Source: CAD feature listing. Evaluate the final solid. Frame: model axes, mm. Face numbers are marked on the shaded views. A direction names the side the tool comes from. Round coordinates to 2 decimals unless told otherwise and drop trailing zeros. Loops run counter-clockwise (first coordinate to the right, second up) from the corner with the lowest first, then second, coordinate; pieces in that order, holes last.
Item 1: Section query B-B on y = -10.5. Return loops of the section in (x, z).
Item 2: First-contact query: P1, Ø1.5, axis at x = 0, y = -1.5, coming from the -Z side. Flat tip, straight axial feed; report the tip coordinate or a pass-through.
Item 3: Access query for the marked faces 1 and 2. Directions: +Z, -Z, +X, -X, +Y, -Y. A direction counts if a zero-diameter tool reaches every point of the face in a straight line with its end or side. Return the directions, or none.
Item 4: Section query A-A on z = 8. Return loops of the section in (x, y) (3 decimals).
Item 5: Section query D-D on y = -7.75. Return loops of the section in (x, z), then the cut area to 3 significant figures.
Item 6: Section query C-C on z = 64. Return loops of the section in (x, y) (3 decimals), then the cut area to 3 significant figures.
Item 7: Pull-direction query (Y, two-part tool) for the marked faces 3, 4 and 5; classes: released by +Y, released by -Y, zero draft, split by the parting line, or undercut.
Item 8: Ray query, L1, parallel to Y at x = -3, z = 12.5 (3 decimals); L2, parallel to X at y = -10.9, z = 8; L3, parallel to X at y = -8, z = 49. Return the intervals inside material, ascending.
```python
from build123d import *

# Parameters (mm, degrees)
SKETCH1_R           = 1.6
BOSS_EXTRUDE1_DEPTH = 2
BOSS_EXTRUDE2_START = 4.6625
BOSS_EXTRUDE2_DEPTH = 4.6625


with BuildPart() as part:
    # Sketch1 → Boss-Extrude1 (new body)
    with BuildSketch(Plane(origin=(0, 0, 0), x_dir=(1, 0, 0), z_dir=(0, 1, 0))):
        with BuildLine():
            Line((-5.70625, 0), (5.70625, 0))
            Line((5.70625, 0), (5.70625, -68))
            ThreePointArc((5.70625, -68), (3.584929656, -67.121320344), (2.70625, -65))
            Line((2.70625, -65), (-5.70625, -10))
            Line((-5.70625, -10), (-5.70625, 0))
        make_face()
        with Locations(Location((-2.70625, -3, 0), (0, 0, 270))):
            Circle(SKETCH1_R, mode=Mode.SUBTRACT)
        with Locations(Location((-2.70625, -8, 0), (0, 0, 270))):
            Circle(SKETCH1_R, mode=Mode.SUBTRACT)
    boss_extrude1 = extrude(amount=BOSS_EXTRUDE1_DEPTH)

    # Sketch2 → Boss-Extrude2 (add)
    with BuildSketch(Plane.XZ.offset(BOSS_EXTRUDE2_START)):
        with BuildLine():
            Line((5.70625, 68), (5.70625, 0))
            Line((5.70625, 0), (2.70625, 0))
            Line((2.70625, 0), (2.70625, 65))
            ThreePointArc((2.70625, 65), (3.584929656, 67.121320344), (5.70625, 68))
        make_face()
    boss_extrude2 = extrude(amount=-BOSS_EXTRUDE2_DEPTH)

    # Mirror6: Boss-Extrude2 across plane
    add(boss_extrude2.mirror(Plane(origin=(0, -4.6625, 0), x_dir=(0, 0, 1), z_dir=(0, -1, 0))))

    # Mirror7: Boss-Extrude1 across plane
    add(boss_extrude1.mirror(Plane(origin=(0, -4.6625, 0), x_dir=(0, 0, 1), z_dir=(0, -1, 0))))


solid = part.part
```
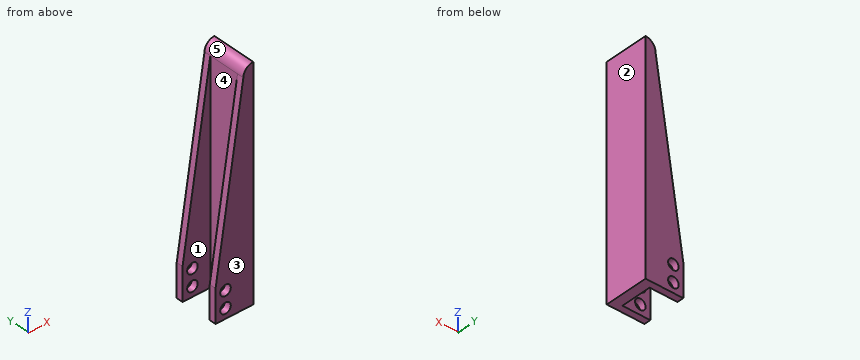
Data:
1. outline: (-5.71, 0) - (5.71, 0) - (5.71, 68) arc R3 ccw to (2.71, 65) - (-5.71, 10) - close; hole circle Ø3.2 at (-2.71, 3); hole circle Ø3.2 at (-2.71, 8)
2. P1: passes through
3. face 1: +Z, -Z, -X
3. face 2: +Z, -Z, +X, +Y, -Y
4. outline: (-5.706, -11.325) - (-4.306, -11.325) - (-4.306, -9.325) - (-5.706, -9.325) - close; (-5.706, 0) - (-4.306, 0) - (-4.306, 2) - (-5.706, 2) - close; (-1.106, -11.325) - (5.706, -11.325) - (5.706, 2) - (-1.106, 2) - (-1.106, 0) - (2.706, 0) - (2.706, -9.325) - (-1.106, -9.325) - close
5. outline: (2.71, 0) - (5.71, 0) - (5.71, 68) arc R3 ccw to (2.71, 65) - close
5. area: 202 mm2
6. outline: (2.553, -11.325) - (5.706, -11.325) - (5.706, 2) - (2.553, 2) - (2.553, 0) - (2.706, 0) - (2.706, -9.325) - (2.553, -9.325) - close
6. area: 40.6 mm2
7. face 3: released by -Y
7. face 4: undercut
7. face 5: zero draft
8. L1: y = -11.325 to -9.325, 0 to 2
8. L2: x = -5.71 to -4.31, -1.11 to 5.71
8. L3: x = 2.71 to 5.71
